Source: CAD feature listing. Evaluate the final solid. Frame: model axes, mm. A direction names the side the tool comes from. Give positions to 0.01 mm unless a question says otherwise; leave off trailing zeros. Order: outer loops, then holes, each group sorted by start corner. A loop starts at its lowest first (then second) coordinate and runs counter-clockwise, first axis right, second up. Notation, with made-up numbers: M -22.5,73.25 L 28.5,73.25 A16 cw 28.5,100.25 Z; hole C 84.5,41.25 d7. An arc over 180 degrees is marked long. Answer in a Markdown table with one row per item. Add a question column.
(1) Pin query (flat end, axial travel): P1, Ø1, axis at x = -40, y = -48, coming from the +Z side; P2, Ø8, axis at y = -150.5, z = -81, coming from the -X side; P3, Ø12, axis at x = -84.5, y = -59.5, coming from the +Z side. Return the tip coordinate at first contact, or that it passes through.
(2) Section query C-C, the plane y = -240. Return loops of the section in (x, z), plus the area to 3 significant figures.
(3) Set-up query: faces 1 (the face through (-97.417, -245.247, 8.502)), 2 (the face through (0.262, -245.247, -102.42)). Return all of +Z, -Z, +X, -X, +Y, -Y with unobstructed straight access to the full face (end or side cutting, diameter ignored); none if empty.
(4) Section query A-A, the plane y = -130.5. Return loops of the section in (x, z).
(5) Material intervals for line 1 along X through (y, z) = (-140.5, -48); line 2 along Y through (x, z) = (80, 112.5); line 3 along X through (y, z) = (-114, 114), sorted ascending.
(6) Mould query, pull axis X, two halves, no side actions, for faces 3 (the face through (-5, 0, 12)), 4 (the face through (107.665, -103, 1)), 5 (the face through (77.35, -178.35, 3.75)). Classes: pulls with the +X half, pulls with the -X half, needs draft (parallel to the pull), parting line crosses it, or undercut.
(7) Section query B-B, the plane y = -49. Return loops of the section in (x, z), plus the area to 3 significant figures.
from build123d import *

# Parameters (mm, degrees)
F3_DEPTH = 260.523276
F4_R     = 50.8
F0_R     = 38.1
F1_DEPTH = 285.439702


with BuildPart() as f3:
    # F2 (on Front) → F3 (new body)
    with BuildSketch(Plane.XZ):
        Polygon((-113.660068, 137.07054), (-110.191997, -116.905782), (107.665264, -116.905782), (107.665264, 121.432772), align=None)
    extrude(amount=F3_DEPTH)

    # F4
    f4_edges = [f3.edges().sort_by_distance(p)[0] for p in [
        (-2.997402, -260.523276, 129.251656),
        (-111.926032, -260.523276, 10.082379),
        (-1.263367, -260.523276, -116.905782),
        (107.665264, -260.523276, 2.263495),
    ]]
    fillet(f4_edges, radius=F4_R)

    # F0 (on face) → F1 (cut)
    with BuildSketch(Plane(origin=(0, 0, -116.905782), x_dir=(1, 0, 0), z_dir=(0, 0, -1))):
        with Locations((56.865264, 146.223276)):
            Circle(F0_R)
    extrude(amount=-F1_DEPTH, mode=Mode.SUBTRACT)


solid = f3.part
Values follow:
| question | item | result |
|---|---|---|
| 1 | P1 | stops at z = 131.9 |
| 1 | P2 | stops at x = -110.74 |
| 1 | P3 | stops at z = 135.43 |
| 2 | outline | M -103.5,126.32 L -100.32,-106.9 L 97.66,-106.9 L 97.66,112.11 Z |
| 2 | area | 45,100 mm² |
| 3 | face 1 | -Z, -X, -Y |
| 3 | face 2 | -Z, +X, -X, -Y |
| 4 | outline | M -113.66,137.07 L -110.19,-116.91 L 22.16,-116.91 L 22.16,127.47 Z; M 91.57,-116.91 L 107.67,-116.91 L 107.67,121.43 L 91.57,122.57 Z |
| 5 | line 1 | x = -111.13 to 19.2, 94.53 to 107.67 |
| 5 | line 2 | y = -241.12 to -176.5, -115.95 to 0 |
| 5 | line 3 | x = -113.35 to 36.54, 77.19 to 107.67 |
| 6 | face 3 | needs draft |
| 6 | face 4 | pulls with the +X half |
| 6 | face 5 | undercut |
| 7 | outline | M -113.66,137.07 L -110.19,-116.91 L 107.67,-116.91 L 107.67,121.43 Z |
| 7 | area | 54,000 mm² |
